Input: part model. Units: mm. Frame: model coordinates. A direction names the side the tool comes from. Give positions to 0.01 mm unless a question says otherwise; leave off trailing zeros. Loops run counter-clockwise (first coordinate to the right, second up) from the corner with the lowest first, then second, coordinate; pieces in that order, holes last.
from build123d import *

# Parameters (mm, degrees)
CUT_EXTRUDE1_DEPTH = 1.4


with BuildPart() as part:
    # Sketch2 → Revolve1 (revolve)
    with BuildSketch(Plane(origin=(0, 0, 0), x_dir=(0, 0, -1), z_dir=(1, 0, 0)), mode=Mode.PRIVATE) as revolve1_sk:
        with BuildLine():
            Line((-2.825, 0), (2.825, 0))
            Line((2.825, 0), (2.825, 1.1))
            Line((2.825, 1.1), (2.425, 1.5))
            Line((2.425, 1.5), (-1.175, 1.5))
            Line((-1.175, 1.5), (-1.175, 2.85))
            Line((-1.175, 2.85), (-1.4225, 2.85))
            ThreePointArc((-1.4225, 2.85), (-2.22987489, 2.285251969), (-2.825, 1.5))
            Line((-2.825, 1.5), (-2.825, 0))
        make_face()
    revolve(revolve1_sk.sketch.rotate(Axis((0, 0, 2.825), (0, 0, -1)), 90), axis=Axis((0, 0, 2.825), (0, 0, -1)))

    # Sketch3 → Cut-Extrude1 (cut)
    with BuildSketch(Plane.XY.offset(2.825)):
        Polygon((0, 1.154700538), (-1, 0.577350269), (-1, -0.577350269), (0, -1.154700538), (1, -0.577350269), (1, 0.577350269), align=None)
    extrude(amount=-CUT_EXTRUDE1_DEPTH, mode=Mode.SUBTRACT)

    # Cut-Extrude2 cone 1 section (through the dimple's axis) → Cut-Extrude2 (revolve, cut)
    with BuildSketch(Plane(origin=(0, 0, 2.825), x_dir=(0, -1, 0), z_dir=(1, 0, 0))):
        Polygon((0, 0), (1.154700538, 0), (0, 1.154700538), align=None)
    revolve(axis=Axis((0, 0, 2.825), (0, 0, -1)), mode=Mode.SUBTRACT)


solid = part.part
(1) Ray query, probe 1 along X at (y, z) = (-0.1, 2.3); probe 2 along Z at (x, y) = (0.05, -0.2) (3 decimals); probe 3 along X at (y, z) = (1, -0.2). Return the intervals inside material, ascending.
Values follow:
probe 1: x = -2.21 to -1, 1 to 2.21
probe 2: z = -2.825 to 1.425
probe 3: x = -1.12 to 1.12
(2) Cut plane D-D (z = -1.6). Return the cut outline in (x, y).
Values follow:
outline: circle Ø3 at (0, 0)
(3) Reachability of faces 1 (the flat face through (0, 0, -2.825)), 2 (the flat face through (-0.51, -0.86, 2.13)) from +Z, -Z, +X, -X, +Y, -Y: full face, straight path, thin tool, end or side. Return the list, or none.
Values follow:
face 1: -Z, +X, -X, +Y, -Y
face 2: +Z
(4) Cut plane B-B (z = 2.05). Return the cut outline in (x, y).
Values follow:
outline: circle Ø4.89 at (0, 0); hole (-1, -0.58) - (0, -1.15) - (1, -0.58) - (1, 0.58) - (0, 1.15) - (-1, 0.58) - close
(5) Mould query, pull axis X, two halves, no side actions, for faces 3 (the cylindrical face through (1.43, -0.45, -0.6)), 4 (the flat face through (1, 0, 2)), 5 (the flat face through (0, 0, 1.425)), 6 (the flat face through (-1.2, 1.2, 1.175)). Classes: +X half, -X half, draft (parallel to the pull), parting line (faces both ways), or undercut.
Values follow:
face 3: parting line
face 4: undercut
face 5: undercut
face 6: draft
(6) Pin query (flat end, axial travel): pin 1 Ø1.3 at (y, z) = (0.5, 2) entering from +X; pin 2 Ø0.9 at (y, z) = (0, 2.5) entering from -X; pin 3 Ø1 at (x, y) = (0, 0) entering from +Z (3 decimals). Return the tip coordinate at first contact, or that it passes through.
Values follow:
pin 1: stops at x = 2.84
pin 2: stops at x = -2.45
pin 3: stops at z = 1.425
